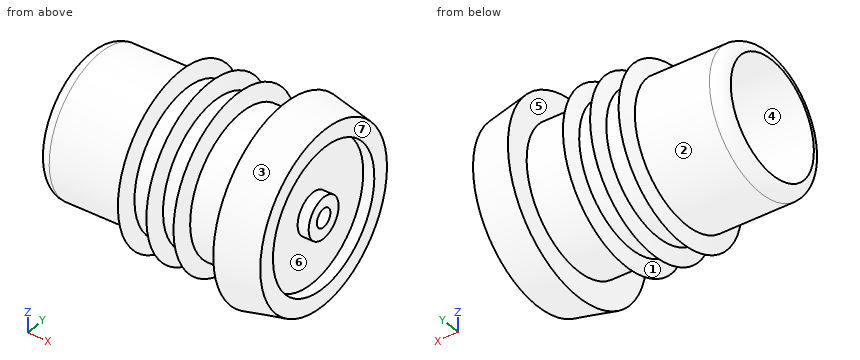
```python
from build123d import *

# Parameters (mm, degrees)
F2_R = 1.5


with BuildPart() as f1:
    # F0 (on Front) → F1 (revolve)
    with BuildSketch(Plane.XZ):
        Polygon((-9.172741, 10.47979), (-9.804832, 8.599592), (-8.490813, 8.599592), align=None)
        Polygon((-5.833726, 10.47979), (-6.465817, 8.599592), (-5.151798, 8.599592), align=None)
        Polygon((-13.314019, 8.599592), (-24, 8.599592), (-24, 7.051038), (1.923128, 7.051038), (1.923128, 1.143372), (5.041865, 1.143372), (5.041865, 2.537624), (3.681099, 2.537624), (3.681099, 8.599592), (5.041865, 8.599592), (5.041865, 10.75), (0, 11.77545), (0, 8.599592), (-5.151798, 8.599592), (-6.465817, 8.599592), (-8.490813, 8.599592), (-9.804832, 8.599592), (-12, 8.599592), align=None)
        Polygon((-12.681928, 10.47979), (-13.314019, 8.599592), (-12, 8.599592), align=None)
    revolve(axis=Axis((-12, 0, 0), (-1, 0, 0)))

    # F2
    f2_edges = [f1.edges().sort_by_distance(p)[0] for p in [
        (-24, 0, -8.599592),
    ]]
    fillet(f2_edges, radius=F2_R)


solid = f1.part
```
For this review, take the finished solid that the model builds, in its own axes (mm). Face numbers are marked on the shaded views. A direction names the side the tool comes from. Coordinates: 2 decimals unless noted, no trailing zeros. Loops run counter-clockwise (first coordinate to the right, second up) from the corner with the lowest first, then second, coordinate; pieces in that order, holes last.
1. Mouldability with a two-part tool opening along X and no side actions: class the marked faces 1, 2 and 3 as +X half, -X half, draft (parallel to the pull), parting line (faces both ways), or undercut.
2. Insertion check: P1, Ø10, axis at y = 7.5, z = -0.5, coming from the -X side; P2, Ø12, axis at x = -14.5, z = -5, coming from the +Y side; P3, Ø5, axis at x = -15, y = -4, coming from the -Z side; P4, Ø12, axis at x = -6.5, z = -2, coming from the -Y side. Each pin has a flat end and moves straight along its axis. Give the tip position at first contact, or say it passes through.
3. Add section A-A, the plane x = -16.75. Give the boundary of the cut face in (y, z), then the cut area to 3 significant figures.
4. Add section B-B, the plane x = 2.75. Give the boundary of the cut face in (y, z), then the cut area to 3 significant figures.
5. For the marked faces 4, 5, 6 and 7, list the 3-axis set-ups (+Z, -Z, +X, -X, +Y, -Y) from which the entire face can be reached by the end or side of a thin tool; tool diameter is ignored.
6. For line 1 (X direction, y = -5.25, z = 7); line 2 (X direction, y = -8.75, z = -2.75); line 3 (Y direction, x = 4.1, z = 0), list the stretches that pass through material, from the lowest coordinate up.
Result:
1. face 1: undercut
1. face 2: draft
1. face 3: +X half
2. P1: stops at x = -24
2. P2: stops at y = 10.48
2. P3: stops at z = -10.02
2. P4: stops at y = -10.48
3. outline: circle Ø17.2 at (0, 0); hole circle Ø14.1 at (0, 0)
3. area: 76.1 mm2
4. outline: circle Ø22.43 at (0, 0); hole circle Ø2.29 at (0, 0)
4. area: 391 mm2
5. face 4: -X
5. face 5: none
5. face 6: +X
5. face 7: +Z, -Z, +X, +Y, -Y
6. line 1: x = -13.26 to -12.05, -9.75 to -8.55, -6.42 to -5.21, 0 to 5.04
6. line 2: x = -13.12 to -12.21, -9.61 to -8.7, -6.27 to -5.36, 0 to 5.04
6. line 3: y = -10.94 to -8.6, -2.54 to -1.14, 1.14 to 2.54, 8.6 to 10.94
